Source: CAD feature listing. Evaluate the final solid. Frame: model axes, mm. A direction names the side the tool comes from. Round coordinates to 2 decimals unless told otherwise and drop trailing zeros. Write each loop counter-clockwise with the first axis right and the second up, starting at its lowest first coordinate (ties: lowest second). Pieces come first, ordered by that corner, then holes.
Autodesk Inventor part; units mm, degrees
ref_plane "YZ Plane" through (0, 0, 0) normal (1, 0, 0) x (0, 1, 0)
ref_plane "XZ Plane" through (0, 0, 0) normal (0, 1, 0) x (-1, 0, 0)
ref_plane "XY Plane" through (0, 0, 0) normal (0, 0, 1) x (1, 0, 0)
sketch "Sketch1" plane through (0, 0, 0) normal (0, 1, 0) x (-1, 0, 0)
  line L0 (15, -15) -> (-15, -15)
  line L1 (-15, -15) -> (-15, 15)
  line L2 (-15, 15) -> (15, 15)
  line L3 (15, 15) -> (15, -15)
  line L4 (15, -15) -> (-15, 15) construction
  line L5 (-15, -15) -> (15, 15) construction
  point P0 (0, 0)
  point P1 (5, 5)
  dimension "d0" = 30
  dimension "d1" = 30
  dimension "d2" = 10
  dimension "d3" = 10
extrude "Extrusion1" add sketch "Sketch1" along normal blind 15
hole "Hole1" at (-5, 0, 5) direction (0, 1, 0) diameter 4.134 end through all counterbore diameter 12.24 counterbore depth 3.58
properties part number "Soporte_Base_Madera" material "PC/ABS Plastic"
1) Pull-direction query (Z, two-part tool) for faces 3 (the face through (15, 7, 0)), 4 (the face through (0, 7, 15)), 5 (the face through (0, 7, -15)), 6 (the face through (-2, 3.58, 5)); classes: released by +Z, released by -Z, zero draft, split by the parting line, or undercut.
Taken from the geometry:
face 3: zero draft
face 4: released by +Z
face 5: released by -Z
face 6: undercut
2) Section query C-C on y = 2.25. Return the cut outline in (x, z).
Taken from the geometry:
outline: (-15, -15) - (15, -15) - (15, 15) - (-15, 15) - close; hole circle Ø12.24 at (-5, 5)
3) Reachability of faces 1 (the face through (-6.838, 1.815, -0.837)), 2 (the face through (-7.05, 9.37, 5.27)) from +Z, -Z, +X, -X, +Y, -Y: full face, straight path, thin tool, end or side. Return the list, or none.
Taken from the geometry:
face 1: -Y
face 2: +Y, -Y
4) Contact query for a flat-ended pin moving along its axis: P1, Ø3.5, axis at x = -3, z = 4, coming from the -Y side. Output: stop coordinate, or through.
Taken from the geometry:
P1: stops at y = 3.58
5) Section query D-D on z = 2. Return the cut outline in (x, y), then the cut area to 3 significant figures.
Taken from the geometry:
outline: (-15, 0) - (-10.33, 0) - (-10.33, 3.58) - (0.33, 3.58) - (0.33, 0) - (15, 0) - (15, 15) - (-15, 15) - close
area: 412 mm2
6) Material intervals for line 1 (X direction, y = 10.75, z = 5); line 2 (X direction, y = 2.45, z = 5); line 3 (Z direction, x = -5, y = 2.4), sorted ascending.
Taken from the geometry:
line 1: x = -15 to -7.07, -2.93 to 15
line 2: x = -15 to -11.12, 1.12 to 15
line 3: z = -15 to -1.12, 11.12 to 15
7) Section query B-B on x = -5. Return the cut outline in (y, z), then the cut area to 3 significant figures.
Taken from the geometry:
outline: (0, -15) - (15, -15) - (15, 2.93) - (3.58, 2.93) - (3.58, -1.12) - (0, -1.12) - close; (0, 11.12) - (3.58, 11.12) - (3.58, 7.07) - (15, 7.07) - (15, 15) - (0, 15) - close
area: 359 mm2
8) Section query A-A on z = 5. Return the cut outline in (x, y), then the cut area to 3 significant figures.
Taken from the geometry:
outline: (-15, 0) - (-11.12, 0) - (-11.12, 3.58) - (-7.07, 3.58) - (-7.07, 15) - (-15, 15) - close; (-2.93, 3.58) - (1.12, 3.58) - (1.12, 0) - (15, 0) - (15, 15) - (-2.93, 15) - close
area: 359 mm2
